Read the model definition and answer for the solid it produces. Units are mm, in the model's axes. Round coordinates to 2 decimals unless told otherwise and drop trailing zeros. Order: outer loops, then holes, each group sorted by start corner. A loop starts at its lowest first (then second) coordinate and runs counter-clockwise, first axis right, second up. Notation, with made-up numbers: (18, 67.5) -> (33, 67.5) arc R27 ccw to (33, 84.5) -> close; hole circle Ø10 at (88.25, 39.5). An arc over 180 degrees is marked (long way). Answer as a JSON object with one key per item and string values. Group by question number.
Item 1: Section A-A, the plane y = -18.8 is taken. Write down the section's boundary in (x, z).
Item 2: Section B-B, the plane x = 0 is taken. Write down the section's boundary in (y, z).
Item 3: Given P1, Ø0.9, axis at x = 35.5, z = 1.5, coming from the +Y side; P2, Ø1.5, axis at y = 39, z = 1, coming from the +X side; P3, Ø1.5, axis at y = 10.5, z = 2, coming from the -X side, each flat-ended and moving along its own axis, determine where each tip first touches the part or whether it passes through.
Item 4: Consider probe 1 along Y at (x, z) = (36.68, 1.65); probe 2 along X at (y, z) = (-27.5, 1.3); probe 3 along Y at (x, z) = (15.5, 0.8). Determine where each line is inside the solid, lowest interval first. Write a range as from..to.
Item 5: Section D-D, the plane z = 0.95 is taken. Count the separate pieces of the cut face and the enclosed holes in it, plus the area to 3 significant figures.
Item 6: Section C-C, the plane y = -27.1 is taken. Write down the section's boundary in (x, z), plus the area to 3 significant figures.
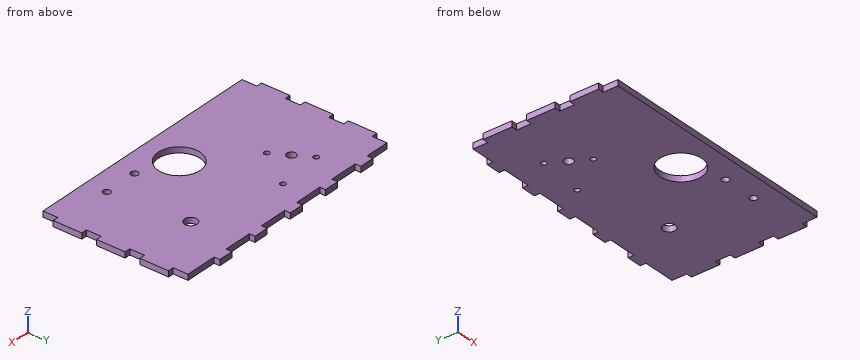
from build123d import *

# Parameters (mm, degrees)
MODEL_R             = 1.397
MODEL_R_2           = 1.89865
MODEL_R_3           = 3.25
MODEL_R_4           = 2.3749
MODEL_R_5           = 11
BOSS_EXTRUDE1_DEPTH = 3


with BuildPart() as part:
    # Model → Boss-Extrude1 (new body)
    with BuildSketch(Plane.XY):
        Polygon((67.32, 30.3), (64.32, 30.3), (64.32, 38.1), (47.48, 38.1), (47.48, 41.1), (39.68, 41.1), (39.68, 38.1), (24.68, 38.1), (24.68, 41.1), (16.88, 41.1), (16.88, 38.1), (1.88, 38.1), (1.88, 41.1), (-5.92, 41.1), (-5.92, 38.1), (-20.92, 38.1), (-20.92, 41.1), (-28.72, 41.1), (-28.72, 38.1), (-43.72, 38.1), (-43.72, 41.1), (-51.52, 41.1), (-51.52, 38.1), (-64.32, 38.1), (-64.32, 30.3), (-67.32, 30.3), (-67.32, 15.3), (-64.32, 15.3), (-64.32, 7.5), (-67.32, 7.5), (-67.32, -7.5), (-64.32, -7.5), (-64.32, -15.3), (-67.32, -15.3), (-67.32, -30.3), (-64.32, -30.3), (-64.32, -38.1), (64.32, -38.1), (64.32, -30.3), (67.32, -30.3), (67.32, -15.3), (64.32, -15.3), (64.32, -7.5), (67.32, -7.5), (67.32, 7.5), (64.32, 7.5), (64.32, 15.3), (67.32, 15.3), align=None)
        with Locations((-37.648489217, 22.560364418)):
            Circle(MODEL_R, mode=Mode.SUBTRACT)
        with Locations((-27.405334652, 4.893459451)):
            Circle(MODEL_R, mode=Mode.SUBTRACT)
        with Locations((-13.343817362, 24.849143198)):
            Circle(MODEL_R, mode=Mode.SUBTRACT)
        with Locations((36.68, -27.1)):
            Circle(MODEL_R_2, mode=Mode.SUBTRACT)
        with Locations((18.68, -27.1)):
            Circle(MODEL_R_2, mode=Mode.SUBTRACT)
        with Locations((32.526911935, 13.726911935)):
            Circle(MODEL_R_3, mode=Mode.SUBTRACT)
        with Locations((-32.526911935, 13.726911935)):
            Circle(MODEL_R_4, mode=Mode.SUBTRACT)
        with Locations((0, -18.8)):
            Circle(MODEL_R_5, mode=Mode.SUBTRACT)
    extrude(amount=BOSS_EXTRUDE1_DEPTH)


solid = part.part
Values found:
{
 "1": {"outline": "(-67.32, 0) -> (-11, 0) -> (-11, 3) -> (-67.32, 3) -> close; (11, 0) -> (67.32, 0) -> (67.32, 3) -> (11, 3) -> close"},
 "2": {"outline": "(-38.1, 0) -> (-29.8, 0) -> (-29.8, 3) -> (-38.1, 3) -> close; (-7.8, 0) -> (41.1, 0) -> (41.1, 3) -> (-7.8, 3) -> close"},
 "3": {"P1": "y = 38.1", "P2": "x = 47.48", "P3": "x = -64.32"},
 "4": {"probe 1": "-38.1..-29, -25.2..38.1", "probe 2": "-67.32..-6.73, 6.73..16.82, 20.54..34.82, 38.54..67.32", "probe 3": "-38.1..38.1"},
 "5": {"separate pieces": "1", "enclosed holes": "8", "area": "9,720 mm2"},
 "6": {"outline": "(-67.32, 0) -> (-7.22, 0) -> (-7.22, 3) -> (-67.32, 3) -> close; (7.22, 0) -> (16.78, 0) -> (16.78, 3) -> (7.22, 3) -> close; (20.58, 0) -> (34.78, 0) -> (34.78, 3) -> (20.58, 3) -> close; (38.58, 0) -> (67.32, 0) -> (67.32, 3) -> (38.58, 3) -> close", "area": "338 mm2"}
}
